Design review of the part built by this model. Coordinates are the model's own, in mm. A direction names the side the tool comes from. Round coordinates to 2 decimals unless told otherwise and drop trailing zeros. Order: outer loops, then holes, each group sorted by start corner. A loop starts at its lowest first (then second) coordinate and runs counter-clockwise, first axis right, second up. Notation, with made-up numbers: (11.5, 43.5) - (53.5, 43.5) arc R21 cw to (53.5, 58.5) - close; hole circle Ø7 at (45, 77.25). An arc over 180 degrees is marked (long way). Use CSV: the item, a comma, the result in double quotes.
Autodesk Inventor part; units mm, degrees
ref_plane "Work Plane1" through (0, 0, 3.5) normal (0, 0, 1) x (1, 0, 0)
ref_plane "YZ Plane" through (0, 0, 0) normal (1, 0, 0) x (0, 1, 0)
ref_plane "XZ Plane" through (0, 0, 0) normal (0, 1, 0) x (-1, 0, 0)
sketch "Sketch1" plane through (0, 0, 0) normal (0, 0, 1) x (1, 0, 0)
  line L0 (0, 0) -> (0, 2)
  line L1 (0, 2) -> (5, 2)
  line L2 (5, 2) -> (5, 3.5)
  line L3 (5, 3.5) -> (20, 3.5)
  line L4 (20, 3.5) -> (20, 5.5)
  line L5 (20, 5.5) -> (21.4643, 5.5)
  line L6 (21.4643, 5.5) -> (21.4643, 5.5)
  line L7 (21.4643, 5.5) -> (24, 5.5)
  line L8 (24, 5.5) -> (24, 2.25)
  line L9 (24, 2.25) -> (40, 2.25)
  line L10 (40, 2.25) -> (40, 3.5)
  line L11 (40, 3.5) -> (47, 3.5)
  line L12 (47, 3.5) -> (47, 0)
  line L13 (47, 0) -> (0, 0)
  dimension "d0" = 4
  dimension "d1" = 7
  dimension "d2" = 5
  dimension "d3" = 15
  dimension "d4" = 47
  dimension "d5" = 7
  dimension "d6" = 16
  dimension "d7" = 4.5
  dimension "d8" = 4
  dimension "d10" = 11
revolve "Revolution1" add sketch "Sketch1" angle 360 about axis through (47, 0, 0) along (-1, 0, 0)
thread "Thread1"
chamfer "Chamfer1" distance 0.5 angle 45 2 edges at (24, -5.5, 0) (47, -3.5, 0)
ref_plane "Work Plane1" through (0, 0, 3.5) normal (0, 0, 1) x (1, 0, 0)
sketch "Sketch2" plane through (0, 0, 3.5) normal (0, 0, 1) x (1, 0, 0)
  line L0 (5, 3.5) -> (5, -3.5)
  point P0 (0, 0)
  point P1 (12.5, 0)
  dimension "d18" = 7.5
hole "Hole1" at (12.5, 0, 3.5) direction (0, 0, -1) diameter 3 end through all
sketch "Sketch4" plane through (0, 0, 0) normal (0, 0, 1) x (1, 0, 0)
  line L0 (44.893, 3.5) -> (42.8722, 0)
  line L1 (46.5, 3.5) -> (44.893, 3.5)
  line L2 (47, 3) -> (47, -3)
  line L3 (46.5, 3.5) -> (40, 3.5)
  line L4 (46.5, -3.5) -> (46.5, 3.5)
  line L5 (46.5, 3.5) -> (44.4793, 0)
  line L6 (44.4793, 0) -> (42.8722, 0)
  point P0 (0, 0)
  point P1 (44.4443, 0)
  point P2 (47, 0)
  point P3 (46.5, 0)
  dimension "d38" = 30
revolve "Revolution3" cut sketch "Sketch4" angle 360 about axis through (44.893, 3.5, 0) along (0.5, 0.8660254, 0)
properties part number "151"
1) The part is to be moulded in two halves that separate along Y. For faces 1 (the face through (14, 0, 0)), 2 (the face through (40, 2.3, 0.7)), 3 (the face through (12.605, 3.233, -1.341)), say which applies: +Y half, -Y half, draft (parallel to the pull), parting line (faces both ways), or undercut.
Data:
face 1,"undercut"
face 2,"draft"
face 3,"parting line"
2) We need section D-D (x = 34). Give the boundary of the cut face in (y, z), then the cut area to 3 significant figures.
Data:
outline,"circle Ø4.5 at (0, 0)"
area,"15.9 mm2"
3) For faces 4 (the face through (32.11, -0.29, 2.23)), 5 (the face through (21.77, -1.19, -5.37)), 6 (the face through (20, 4, 0)), 7 (the face through (43.296, -3.497, 0.154)), list the 3-axis set-ups (+Z, -Z, +X, -X, +Y, -Y) from which the entire face can be reached by the end or side of a thin tool; tool diameter is ignored.
Data:
face 4,"none"
face 5,"+X, -X"
face 6,"-X"
face 7,"+X"
4) We need section C-C (x = 12.5). Give the boundary of the cut face in (y, z), then the cut area to 3 significant figures.
Data:
outline,"(-1.5, -3.16) - (-1.5, 3.16) arc R3.5 ccw to start; (1.5, -3.16) arc R3.5 ccw to (1.5, 3.16) - close"
area,"18.1 mm2"
5) To check wall thickness, follow L1, parallel to X at y = 0, z = 1; L2, parallel to X at y = 2.25, z = 0.5; L3, parallel to Y at x = 12.5, z = 1.75. State the ranges of each line that lie inside material, in increasing order. Write a range as from..to.
Data:
L1,"x = 0..11, 14..47"
L2,"x = 5..24, 40..42.67, 45.67..47"
L3,"y = -3.03..-1.5, 1.5..3.03"
6) We need section B-B (x = 23). Give the boundary of the cut face in (y, z), then the cut area to 3 significant figures.
Data:
outline,"circle Ø11 at (0, 0)"
area,"95.0 mm2"
7) Insertion check: pin 1 Ø2 at (x, z) = (5, 0) entering from -Y; pin 2 Ø1 at (x, z) = (22.5, 2.5) entering from +Y; pin 3 Ø6 at (x, y) = (14, -0.5) entering from +Z. Each pin has a flat end and moves straight along its axis. Give the tip position at first contact, or say it passes through.
Data:
pin 1,"stops at y = -3.5"
pin 2,"stops at y = 5.12"
pin 3,"stops at z = 3.5"
